Could you check a few things on this drawing? It's one solid part, dimensions in mm from its lowest x, y, z. Coordinates: 2 decimals unless noted, no trailing zeros. Write each loop counter-clockwise with the first axis right and the second up, starting at its lowest first coordinate (ties: lowest second). Pieces come first, ordered by that corner, then holes. Notation, with made-up numbers: (81, 31.5) - (85, 31.5) arc R18 cw to (85, 56.5) - close; hole circle Ø7 at (54, 15.5). An arc over 180 degrees is marked (long way). Write item = value, one per line. Start each with the question number.
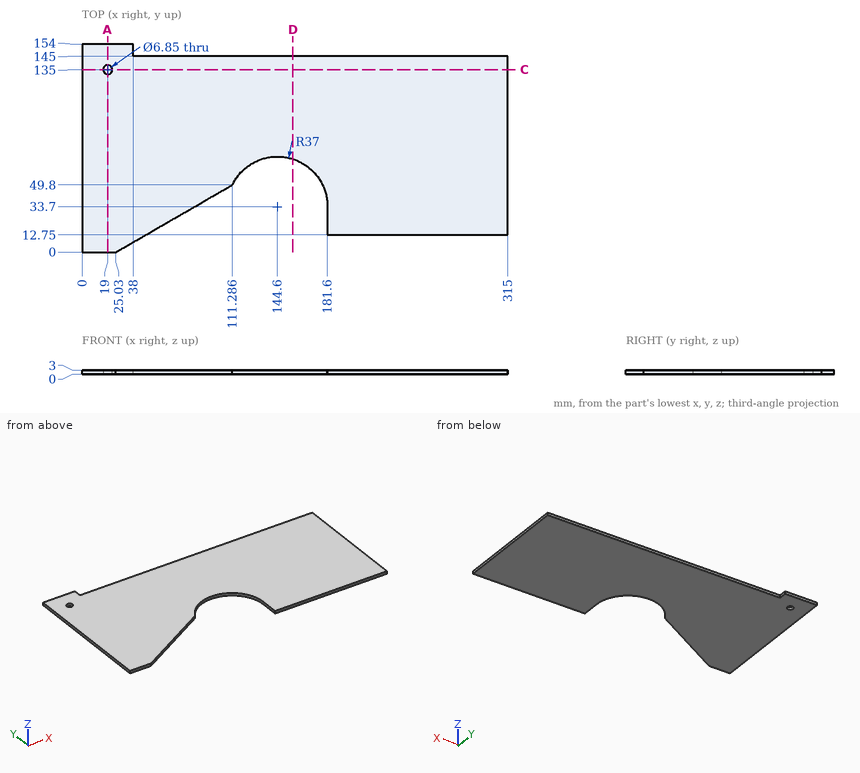
1) Suppose I cut it at D-D on x = 156. Please give me the cut outline in (y, z).
2) For P1, Ø1.5, axis at x = 269.5, z = 2, coming from the -Y side, with a flat end and sliding along its axis, tell me the tip position at first contact or that it passes through.
3) Suppose I cut it at A-A on x = 19. Please give me the cut outline in (y, z) (1 decimal).
4) If I drill on probe 1 along X at (y, z) = (135, 1.5) (1 decimal); probe 2 along Y at (x, z) = (19, 1.15) (1 decimal); probe 3 along Y at (x, z) = (266.5, 1.7), over which ranges is the centre line in solid material (lowest first)? Write a range as [from, to].
5) Suppose I cut it at C-C on y = 135. Please give me the cut outline in (x, z) (1 decimal).
Reply:
q1.outline = (68.9, 0) - (145, 0) - (145, 3) - (68.9, 3) - close
q2.P1 = 12.75
q3.outline = (0, 0) - (131.6, 0) - (131.6, 3) - (0, 3) - close; (138.4, 0) - (154, 0) - (154, 3) - (138.4, 3) - close
q4.probe_1 = [0, 15.6], [22.4, 315]
q4.probe_2 = [0, 131.6], [138.4, 154]
q4.probe_3 = [12.75, 145]
q5.outline = (0, 0) - (15.6, 0) - (15.6, 3) - (0, 3) - close; (22.4, 0) - (315, 0) - (315, 3) - (22.4, 3) - close
